Build history of the part. All positions in model axes, mm. A direction names the side the tool comes from. Coordinates: 2 decimals unless noted, no trailing zeros. Write each loop counter-clockwise with the first axis right and the second up, starting at its lowest first coordinate (ties: lowest second). Pieces come first, ordered by that corner, then holes.
```python
from build123d import *

# Parameters (mm, degrees)
SKETCH1_W                      = 50
SKETCH1_H                      = 80
BOSS_EXTRUDE1_DEPTH            = 10
SKETCH2_W                      = 5
SKETCH2_H                      = 80
BOSS_EXTRUDE2_DEPTH            = 50
SKETCH3_R                      = 12.5
CUT_EXTRUDE1_DEPTH             = 88.749643874
M3_CLEARANCE_HOLE1_D           = 3.4
CBORE_FOR_M5_SHCS1_D           = 5.5
CBORE_FOR_M5_SHCS1_CBORE_D     = 10
CBORE_FOR_M5_SHCS1_CBORE_DEPTH = 5
FILLET11_R                     = 2
BOSS_EXTRUDE3_DEPTH            = 5.08


with BuildPart() as part:
    # Sketch1 → Boss-Extrude1 (new body)
    with BuildSketch(Plane.XY):
        Rectangle(SKETCH1_W, SKETCH1_H)
    extrude(amount=BOSS_EXTRUDE1_DEPTH)

    # Sketch2 → Boss-Extrude2 (add)
    with BuildSketch(Plane.XY.offset(10)):
        with Locations((22.5, 0)):
            Rectangle(SKETCH2_W, SKETCH2_H)
    extrude(amount=BOSS_EXTRUDE2_DEPTH)

    # Sketch3 → Cut-Extrude1 (cut, through all)
    with BuildSketch(Plane(origin=(25, 0, 0), x_dir=(0, 0, -1), z_dir=(1, 0, 0))):
        with Locations((-35, 0)):
            Circle(SKETCH3_R)
    extrude(amount=-CUT_EXTRUDE1_DEPTH, mode=Mode.SUBTRACT)

    # M3 Clearance Hole1 (through all)
    with Locations(Plane(origin=(25, 0, 0), x_dir=(0, 0, -1), z_dir=(1, 0, 0))):
        with Locations((-50.5, -15.5), (-35, 0), (-50.5, 15.5), (-19.5, -15.5), (-19.5, 15.5)):
            Hole(M3_CLEARANCE_HOLE1_D / 2)

    # CBORE for M5 SHCS1 (through all)
    with Locations(Plane.XY.offset(10)):
        with Locations((-15.902931391, 24.76), (10.902931391, 24.76), (-15.902931391, -24.76), (10.902931391, -24.76)):
            CounterBoreHole(CBORE_FOR_M5_SHCS1_D / 2, CBORE_FOR_M5_SHCS1_CBORE_D / 2, CBORE_FOR_M5_SHCS1_CBORE_DEPTH)

    # Fillet11
    fillet11_edges = [part.edges().sort_by_distance(p)[0] for p in [
        (20, 0, 10),
    ]]
    fillet(fillet11_edges, radius=FILLET11_R)

    # Sketch8 → Boss-Extrude3 (add)
    with BuildSketch(Plane.XZ.offset(40)):
        Polygon((20, 60), (-25, 10), (20, 10), align=None)
    extrude(amount=-BOSS_EXTRUDE3_DEPTH)


solid = part.part
```
1. Saw through at C-C on y = -15.5. List the corners of the cut face in (x, z), plus the area to 3 significant figures.
Computed values:
outline: (-25, 0) - (25, 0) - (25, 17.8) - (20, 17.8) - (20, 12) arc R2 cw to (18, 10) - (-25, 10) - close; (20, 21.2) - (25, 21.2) - (25, 48.8) - (20, 48.8) - close; (20, 52.2) - (25, 52.2) - (25, 60) - (20, 60) - close
area: 717 mm2
2. 3-axis set-ups, long thin cutter, end or side, ignore diameter. For faces 1 (the face through (-19.871, -27.802, 7.535)), 2 (the face through (7, -34.92, 24)), 3 (the face through (-2.185, -37.496, 35.35)): which of +Z, -Z, +X, -X, +Y, -Y reach the whole face in a straight line?
Computed values:
face 1: +Z
face 2: +Z, -X, +Y
face 3: +Z, -X, +Y, -Y
3. Probe line 1 along X through (y, z) = (25, 3.5); line 2 along X through (y, z) = (24, 7); line 3 along Y through (x, z) = (17, 46.5). List the from-to ranges inside material, lowest first.
Computed values:
line 1: x = -25 to -18.64, -13.16 to 8.16, 13.64 to 25
line 2: x = -25 to -20.84, -10.96 to 5.96, 15.84 to 25
line 3: y = -40 to -34.92
4. Saw through at D-D on z = 35. List the corners of the cut face in (x, y).
Computed values:
outline: (-2.5, -40) - (25, -40) - (25, -12.5) - (20, -12.5) - (20, -34.92) - (-2.5, -34.92) - close; (20, 12.5) - (25, 12.5) - (25, 40) - (20, 40) - close
5. Mould opens along Z. For faces 4 (the face through (22.47, -15.43, 48.8)), 5 (the face through (20, 10, 46)), 6 (the face through (13, -27, 5)) say: +Z half, -Z half, draft (parallel to the pull), parting line (faces both ways), or undercut.
Computed values:
face 4: undercut
face 5: draft
face 6: +Z half
6. Flat gauge pins, fed straight in: pin 1 (5 mm diameter, centred on x = 10, y = -23.5, fed in from +Z); pin 2 (8 mm diameter, centred on y = 13.5, z = 20.5, fed in from -X); pin 3 (3 mm diameter, centred on x = 5.5, y = -27.5, fed in from +Z). Where does each tip first touch, or does it go through?
Computed values:
pin 1: stops at z = 5
pin 2: stops at x = 20
pin 3: stops at z = 10
7. Saw through at A-A on z = 50.5. List the corners of the cut face in (x, y).
Computed values:
outline: (11.45, -40) - (25, -40) - (25, -17.2) - (20, -17.2) - (20, -34.92) - (11.45, -34.92) - close; (20, -13.8) - (25, -13.8) - (25, 13.8) - (20, 13.8) - close; (20, 17.2) - (25, 17.2) - (25, 40) - (20, 40) - close
8. Saw through at B-B on y = 0. List the corners of the cut face in (x, z).
Computed values:
outline: (-25, 0) - (25, 0) - (25, 22.5) - (20, 22.5) - (20, 12) arc R2 cw to (18, 10) - (-25, 10) - close; (20, 47.5) - (25, 47.5) - (25, 60) - (20, 60) - close
